Read the model definition and answer for the solid it produces. Units are mm, in the model's axes. Give positions to 0.01 mm unless a question says otherwise; leave off trailing zeros. Order: outer loops, then holes, each group sorted by start corner. A loop starts at its lowest first (then second) coordinate and runs counter-clockwise, first axis right, second up. Notation, with made-up numbers: (-9, 11.5) - (43, 11.5) arc R26 cw to (43, 47.5) - close; hole circle Ø2 at (82.25, 30.5). An arc over 180 degrees is marked (long way). Write item = value, one per line.
Autodesk Inventor part; units mm, degrees
ref_plane "YZ Plane" through (0, 0, 0) normal (1, 0, 0) x (0, 1, 0)
ref_plane "XZ Plane" through (0, 0, 0) normal (0, 1, 0) x (-1, 0, 0)
ref_plane "XY Plane" through (0, 0, 0) normal (0, 0, 1) x (1, 0, 0)
sketch "Sketch1" plane through (0, 0, 0) normal (1, 0, 0) x (0, 1, 0)
  line L0 (0, 0) -> (83.185, 0)
  line L1 (83.185, 0) -> (83.185, -50.8)
  line L2 (83.185, -50.8) -> (0, -50.8)
  line L3 (0, -50.8) -> (0, 0)
  circle A0 centre (57.785, -25.4) radius 19.685
  circle A1 centre (14.2875, -14.2875) radius 7.9375
  circle A2 centre (14.2875, -36.5125) radius 7.9375
  circle A3 centre (5.08, -5.08) radius 1.7145
  circle A4 centre (5.08, -45.72) radius 1.7145
  circle A5 centre (78.105, -5.08) radius 1.7145
  circle A6 centre (78.105, -45.72) radius 1.7145
  line L4 (83.185, 0) -> (32.385, 0)
  circle A7 centre (37.465, -47.625) radius 1.7145
  circle A8 centre (37.465, -3.175) radius 1.7145
  circle A9 centre (57.785, -25.4) radius 24.13
  dimension "d0" = 83.185
  dimension "d1" = 50.8
  dimension "d2" = 39.37
  dimension "d3" = 25.4
  dimension "d4" = 25.4
  dimension "d5" = 15.875
  dimension "d6" = 15.875
  dimension "d7" = 14.2875
  dimension "d8" = 14.2875
  dimension "d9" = 14.2875
  dimension "d10" = 14.2875
  dimension "d16" = 3.429
  dimension "d17" = 5.08
  dimension "d18" = 5.08
  dimension "d19" = 50.8
  dimension "d20" = 3.429
  dimension "d21" = 3.175
  dimension "d23" = 48.26
  dimension "d32" = 5.08
  dimension "d33" = 5.08
  dimension "d34" = 3.175
  dimension "d35" = 5.08
  dimension "d36" = 5.08
  dimension "d37" = 5.08
  dimension "d38" = 5.08
extrude "Extrusion1" add sketch "Sketch1" along normal blind 6.35 contours L0 L1 L2 L3 | A9
draft "FaceDraft1" angle 16 pull direction (1, 0, 0) faces at (4.2333, 22.1993, -37.1512) (4.2333, 22.1993, -14.9262) fixed edges at (6.35, 6.35, -36.5125) (6.35, 6.35, -14.2875)
extrude "Extrusion2" add sketch "Sketch1" against normal blind 35.814 contours A9
chamfer "Chamfer1" distance 2.54 angle 20 1 edges at (6.35, 38.1, -25.4) measured on face at (-7.7047, 77.4062, -26.984)
chamfer "Chamfer2" distance 2.54 angle 20 1 edges at (-35.814, 38.1, -25.4) measured on face at (-9.398, 77.2151, -28.5577)
properties part number "Engine Head Bottom"
1. Determine the mould class of faces 1 (the face through (3, 83.185, -25)), 2 (the face through (-17.66, 33.68, -24.34)), 3 (the face through (1.103, 9.183, -40.427)) for opening direction Y: +Y half, -Y half, draft (parallel to the pull), parting line (faces both ways), or undercut.
Recorded:
face_1 = +Y half
face_2 = parting line
face_3 = undercut
2. Section C-C (z = -34) is taken. Count the separate pieces of the cut face and the enclosed holes in it, and give its area (3 significant figures).
Recorded:
separate_pieces = 3
enclosed_holes = 0
area = 561 mm^2
3. Section B-B (x = -10) is taken. Determine the outline of the cut face in (y, z) (3 decimals), and give its area (3 significant figures).
Recorded:
outline = circle Ø48.26 at (57.785, -25.4); hole circle Ø39.37 at (57.785, -25.4)
area = 612 mm^2
4. Straight lines are drawn through the part: L1, parallel to Z at x = 3, y = 5.08; L2, parallel to Y at x = -3, z = -25; L3, parallel to Y at x = 2, z = -41 (3 decimals). For each, find the intervals that lie inside material, in ascending order. Write a range as [from, to].
Recorded:
L1 = [-50.8, -47.43], [-44.01, -6.79], [-3.37, 0]
L2 = [33.66, 38.1], [77.47, 81.91]
L3 = [0, 9.326], [19.249, 45.779], [69.791, 83.185]
5. Flat-ended cylindrical pins translate along their axes: pin 1 (3 mm diameter, centred on y = 37.465, z = -3.175, fed in from +X); pin 2 (10 mm diameter, centred on y = 9.5, z = -34, fed in from -X); pin 3 (12 mm diameter, centred on x = -21, z = -7.5, fed in from +Y); pin 4 (12 mm diameter, centred on x = -18.5, z = -23, fed in from -Y) (3 decimals). Find the tip coordinate at first contact, or state that the pin passes through.
Recorded:
pin_1 = through
pin_2 = 0
pin_3 = 78.78
pin_4 = 33.655
6. Section A-A (z = -25.4) is taken. Determine the outline of the cut face in (x, y) (3 decimals).
Recorded:
outline = (-35.814, 33.655) - (0, 33.655) - (0, 0) - (6.35, 0) - (6.35, 37.176) - (3.81, 38.1) - (-33.274, 38.1) - (-35.814, 37.176) - close; (-35.814, 78.394) - (-33.274, 77.47) - (3.81, 77.47) - (6.35, 78.394) - (6.35, 83.185) - (0, 83.185) - (0, 81.915) - (-35.814, 81.915) - close
